from build123d import *

# Parameters (mm, degrees)
SKETCH1_R                = 2.38125
BOSS_EXTRUDE1_DEPTH      = 231.775
BOSS_EXTRUDE1_DEPTH_BACK = 231.775


with BuildPart() as part:
    # Sketch1 → Boss-Extrude1 (new body, two sides)
    with BuildSketch(Plane(origin=(0, 0, 0), x_dir=(0, 0, -1), z_dir=(1, 0, 0))) as boss_extrude1_sk:
        with BuildLine():
            Line((7.039054482, 0.508), (3.959468146, 5.842))
            ThreePointArc((3.959468146, 5.842), (3.587586336, 6.21388181), (3.079586336, 6.35))
            Line((3.079586336, 6.35), (-3.079586336, 6.35))
            ThreePointArc((-3.079586336, 6.35), (-3.587586336, 6.21388181), (-3.959468146, 5.842))
            Line((-3.959468146, 5.842), (-7.039054482, 0.508))
            ThreePointArc((-7.039054482, 0.508), (-7.175172672, 0), (-7.039054482, -0.508))
            Line((-7.039054482, -0.508), (-3.959468146, -5.842))
            ThreePointArc((-3.959468146, -5.842), (-3.587586336, -6.21388181), (-3.079586336, -6.35))
            Line((-3.079586336, -6.35), (3.079586336, -6.35))
            ThreePointArc((3.079586336, -6.35), (3.587586336, -6.21388181), (3.959468146, -5.842))
            Line((3.959468146, -5.842), (7.039054482, -0.508))
            ThreePointArc((7.039054482, -0.508), (7.175172672, 0), (7.039054482, 0.508))
        make_face()
        Circle(SKETCH1_R, mode=Mode.SUBTRACT)
    extrude(amount=BOSS_EXTRUDE1_DEPTH)
    extrude(boss_extrude1_sk.sketch, amount=-BOSS_EXTRUDE1_DEPTH_BACK)


solid = part.part
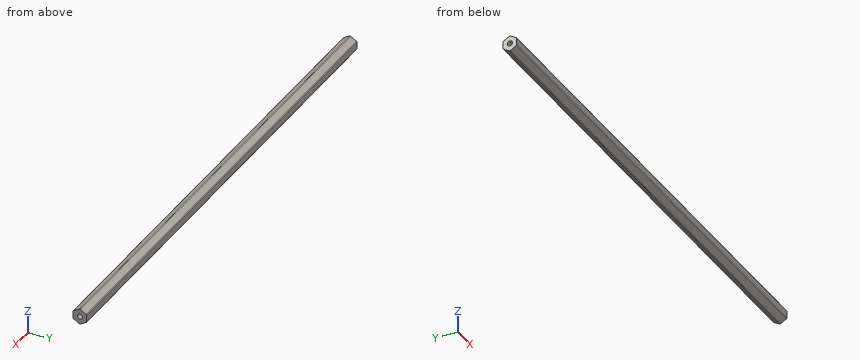
Verification items for the finished model (mm, model axes). Give positions to 0.01 mm unless a question says otherwise; leave off trailing zeros. Order: outer loops, then holes, each group sorted by start corner. A loop starts at its lowest first (then second) coordinate and runs counter-clockwise, first axis right, second up. Notation, with made-up numbers: M 53.5,11 L 73.5,11 A4 ccw 73.5,15 Z; hole C 54,16 d9. An arc over 180 degrees is marked long. Use one line per item in the form item = value. Start each with the question number.
Q1. Scan lines: line 1 along Y through (x, z) = (-75.5, 0); line 2 along Y through (x, z) = (-12, 3.25); line 3 along Z through (x, y) = (-205, 2). Record each from-to range of solid material in increasing order. Write a range as [from, to].
Q2. Section check A-A (x = 37.5). Enter the section's corners in (y, z), then the cut area to 3 significant figures.
Q3. Section check B-B (z = 0). Enter the section's corners in (x, y) (3 decimals).
Q4. Go/stop test with flat-tipped pins: pin 1 Ø4.5 at (y, z) = (0, 0) entering from -X; pin 2 Ø5 at (x, y) = (176, -4.5) entering from +Z; pin 3 Ø1 at (x, z) = (75.5, 4.5) entering from +Y; pin 4 Ø5 at (x, y) = (96, -4) entering from +Z. Record where each tip stops, or that it passes through.
Evaluation:
q1.line_1 = [-6.35, -2.38], [2.38, 6.35]
q1.line_2 = [-6.34, 6.34]
q1.line_3 = [-6.18, -1.29], [1.29, 6.18]
q2.outline = M -6.35,-3.08 A1.02 ccw -5.84,-3.96 L -0.51,-7.04 A1.02 ccw 0.51,-7.04 L 5.84,-3.96 A1.02 ccw 6.35,-3.08 L 6.35,3.08 A1.02 ccw 5.84,3.96 L 0.51,7.04 A1.02 ccw -0.51,7.04 L -5.84,3.96 A1.02 ccw -6.35,3.08 Z; hole C 0,0 d4.76
q2.area = 122 mm2
q3.outline = M -231.775,-6.35 L 231.775,-6.35 L 231.775,-2.381 L -231.775,-2.381 Z; M -231.775,2.381 L 231.775,2.381 L 231.775,6.35 L -231.775,6.35 Z
q4.pin_1 = through
q4.pin_2 = 6.18
q4.pin_3 = 5.77
q4.pin_4 = 6.47
